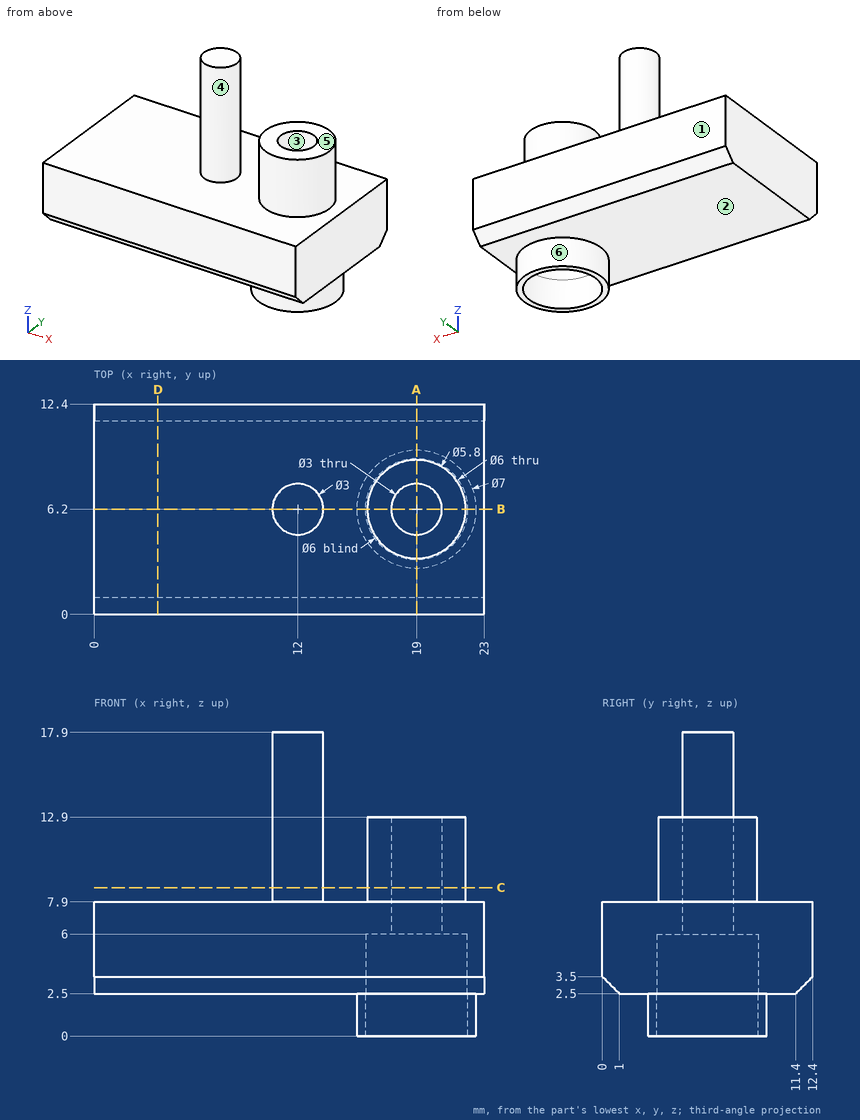
Source: three-view drawing plus pictorial views. Frame: mm from the lowest corner of the part. A direction names the side the tool comes from. Round coordinates to 2 decimals unless told otherwise and drop trailing zeros. Loops run counter-clockwise (first coordinate to the right, second up) from the corner with the lowest first, then second, coordinate; pieces in that order, holes last. Notation, with made-up numbers: M 7.5,-8.5 L 62.5,-8.5 A19 ccw 62.5,0.5 Z; hole C -14.75,55.25 d7. An arc over 180 degrees is marked long. Answer as CSV lines item,"result". Start each with the question number.
(1) Section D-D, the plane x = 3.75. Output: boundary loops of the cut face in (y, z).
(2) Reachability of the marked faces 4, 5 and 6 from +Z, -Z, +X, -X, +Y, -Y: full face, straight path, thin tool, end or side. Return the list, or none.
(3) Draft query along Y for the marked faces 1, 2 and 3. Return one class per face: released by +Y, released by -Y, zero draft, split by the parting line, or undercut.
(4) Section C-C, the plane z = 8.75. Output: boundary loops of the cut face in (x, y), plus the area to 3 significant figures.
(5) First-contact query: pin 1 (2.5 mm diameter, centred on x = 19, y = 6.2, fed in from +Z); pin 2 (3 mm diameter, centred on x = 20.5, z = 10, fed in from +Y); pin 3 (1.5 mm diameter, centred on y = 7, z = 12.5, fed in from +X); pin 4 (5 mm diameter, centred on x = 19, y = 6.2, fed in from +Z). Flat tips, straight axial feed; report the tip coordinate or a pass-through.
(6) Section A-A, the plane x = 19. Output: boundary loops of the cut face in (y, z), plus the area to 3 significant figures.
(7) Line query: line 1 (Y direction, x = 19, z = 1.15); line 2 (Z direction, x = 16.75, y = 9.5); line 3 (X direction, y = 6.2, z = 5.25). Output: solid intervals per line, ascending. Write a range as [from, to].
(8) Section B-B, the plane y = 6.2. Output: boundary loops of the cut face in (x, z).
Values found:
1,outline,"M 0,3.5 L 1,2.5 L 11.4,2.5 L 12.4,3.5 L 12.4,7.9 L 0,7.9 Z"
2,face 4,"+Z"
2,face 5,"+Z, +X, +Y, -Y"
2,face 6,"-Z"
3,face 1,"released by +Y"
3,face 2,"zero draft"
3,face 3,"undercut"
4,outline,"C 12,6.2 d3; C 19,6.2 d5.8; hole C 19,6.2 d3"
4,area,"26.4 mm²"
5,pin 1,"passes through"
5,pin 2,"stops at y = 9.1"
5,pin 3,"stops at x = 21.9"
5,pin 4,"stops at z = 12.9"
6,outline,"M 0,3.5 L 1,2.5 L 2.7,2.5 L 2.7,0 L 3.2,0 L 3.2,6 L 4.7,6 L 4.7,12.9 L 3.3,12.9 L 3.3,7.9 L 0,7.9 Z; M 7.7,6 L 9.2,6 L 9.2,0 L 9.7,0 L 9.7,2.5 L 11.4,2.5 L 12.4,3.5 L 12.4,7.9 L 9.1,7.9 L 9.1,12.9 L 7.7,12.9 Z"
6,area,"55.8 mm²"
7,line 1,"y = [2.7, 3.2], [9.2, 9.7]"
7,line 2,"z = [2.5, 7.9]"
7,line 3,"x = [0, 16], [22, 23]"
8,outline,"M 0,2.5 L 15.5,2.5 L 15.5,0 L 16,0 L 16,6 L 17.5,6 L 17.5,12.9 L 16.1,12.9 L 16.1,7.9 L 13.5,7.9 L 13.5,17.9 L 10.5,17.9 L 10.5,7.9 L 0,7.9 Z; M 20.5,6 L 22,6 L 22,0 L 22.5,0 L 22.5,2.5 L 23,2.5 L 23,7.9 L 21.9,7.9 L 21.9,12.9 L 20.5,12.9 Z"
